from build123d import *

# Parameters (mm, degrees)
SKETCH1_R           = 25
BOSS_EXTRUDE1_DEPTH = 10
FILLET1_R           = 10
BOSS_EXTRUDE2_DEPTH = 3.6
SKETCH3_W           = 3
SKETCH3_H           = 8
BOSS_EXTRUDE3_DEPTH = 27
SKETCH4_R           = 2.4
CUT_EXTRUDE1_DEPTH  = 49.830420846
FILLET2_R           = 4
FILLET3_R           = 1


with BuildPart() as part:
    # Sketch1 → Boss-Extrude1 (new body)
    with BuildSketch(Plane(origin=(0, 0, 0), x_dir=(1, 0, 0), z_dir=(0, 1, 0))):
        with Locations(Location((0, 0, 0), (0, 0, 270))):
            Circle(SKETCH1_R)
    extrude(amount=BOSS_EXTRUDE1_DEPTH)

    # Fillet1
    fillet1_edges = [part.edges().sort_by_distance(p)[0] for p in [
        (0, 10, -25),
    ]]
    fillet(fillet1_edges, radius=FILLET1_R - 0.0001)  # a hair under: the kernel refuses the full size

    # Sketch2 → Boss-Extrude2 (add)
    with BuildSketch(Plane(origin=(0, 10, 0), x_dir=(1, 0, 0), z_dir=(0, 1, 0))):
        with BuildLine():
            Line((-2.226875614, -0.895), (-0.895, -0.895))
            Line((-0.895, -0.895), (-0.895, -2.226875614))
            ThreePointArc((-0.895, -2.226875614), (0, -2.4), (0.895, -2.226875614))
            Line((0.895, -2.226875614), (0.895, -0.895))
            Line((0.895, -0.895), (2.226875614, -0.895))
            ThreePointArc((2.226875614, -0.895), (2.4, 0), (2.226875614, 0.895))
            Line((2.226875614, 0.895), (0.895, 0.895))
            Line((0.895, 0.895), (0.895, 2.226875614))
            ThreePointArc((0.895, 2.226875614), (0, 2.4), (-0.895, 2.226875614))
            Line((-0.895, 2.226875614), (-0.895, 0.895))
            Line((-0.895, 0.895), (-2.226875614, 0.895))
            ThreePointArc((-2.226875614, 0.895), (-2.4, 0), (-2.226875614, -0.895))
        make_face()
    extrude(amount=BOSS_EXTRUDE2_DEPTH)

    # Sketch3 → Boss-Extrude3 (add)
    with BuildSketch(Plane.XZ):
        with Locations((-5.6, 0)):
            Rectangle(SKETCH3_W, SKETCH3_H)
        with Locations((5.6, 0)):
            Rectangle(SKETCH3_W, SKETCH3_H)
    extrude(amount=-BOSS_EXTRUDE3_DEPTH)

    # Sketch4 → Cut-Extrude1 (cut, through all)
    with BuildSketch(Plane(origin=(7.1, 0, 0), x_dir=(0, 0, -1), z_dir=(1, 0, 0))):
        with Locations((0, 23)):
            Circle(SKETCH4_R)
    extrude(amount=-CUT_EXTRUDE1_DEPTH, mode=Mode.SUBTRACT)

    # Fillet2
    fillet2_edges = [part.edges().sort_by_distance(p)[0] for p in [
        (5.6, 27, -4),
        (5.6, 27, 4),
        (-5.6, 27, 4),
        (-5.6, 27, -4),
    ]]
    fillet(fillet2_edges, radius=FILLET2_R - 0.0001)  # a hair under: the kernel refuses the full size

    # Fillet3
    fillet3_edges = [part.edges().sort_by_distance(p)[0] for p in [
        (-7.1, 10, 0),
        (-5.6, 10, 4),
        (-5.6, 10, -4),
        (5.6, 10, 4),
        (7.1, 10, 0),
        (5.6, 10, -4),
    ]]
    fillet(fillet3_edges, radius=FILLET3_R)


solid = part.part
Verification items for the finished model (mm, model axes). A direction names the side the tool comes from. Give positions to 0.01 mm unless a question says otherwise; leave off trailing zeros. Write each loop counter-clockwise with the first axis right and the second up, starting at its lowest first coordinate (ties: lowest second). Pieces come first, ordered by that corner, then holes. Notation, with made-up numbers: M 81,49.5 L 132,49.5 A10 ccw 132,65.5 Z; hole C 39.5,26 d1. An arc over 180 degrees is marked long. Put each result on its own line as item: value. Start each with the question number.
1. Draft check along X on faces 1 (the face through (5.621, 25.797, -2.859)), 2 (the face through (2, 12, -0.895)), 3 (the face through (-2, 12, -0.895)). Enter one of: +X half, -X half, draft (parallel to the pull), parting line (faces both ways), or undercut.
2. Section check C-C (y = 2). Record the cut outline in (x, z), and give its area (3 significant figures).
3. Scan lines: line 1 along Y through (x, z) = (-5, 0); line 2 along X through (y, z) = (14, 2.5); line 3 along Y through (x, z) = (11.5, -2). Record each from-to range of solid material in increasing order. Write a range as [from, to].
4. Section check A-A (y = 18.5). Record the cut outline in (x, z).
5. Go/stop test with flat-tipped pins: pin 1 Ø1 at (x, z) = (7, -16.5) entering from +Y; pin 2 Ø0.9 at (x, y) = (-6, 20) entering from +Z; pin 3 Ø1.1 at (x, y) = (-1.5, 11) entering from +Z (3 decimals). Record where each tip stops, or that it passes through.
6. Set-up check for faces 4 (the face through (0.895, 12, -2)), 5 (the face through (0, 11.8, 2.4)), 6 (the face through (-4.1, 16, 0)), 7 (the face through (2.4, 11.8, 0)), 8 (the face through (-6, 17, 4)): record each of +Z, -Z, +X, -X, +Y, -Y from which the full face is reachable in a straight line by a thin tool's end or side.
Answer list:
1. face 1: draft
1. face 2: undercut
1. face 3: undercut
2. outline: C 0,0 d49.6
2. area: 1,930 mm2
3. line 1: [0, 20.6], [25.4, 27]
3. line 2: [-7.1, -4.1], [4.1, 7.1]
3. line 3: [0, 10]
4. outline: M -7.1,-4 L -4.1,-4 L -4.1,4 L -7.1,4 Z; M 4.1,-4 L 7.1,-4 L 7.1,4 L 4.1,4 Z
5. pin 1: y = 9.7
5. pin 2: z = 4
5. pin 3: z = 0.895
6. face 4: -Z, +Y
6. face 5: +Z, +Y
6. face 6: +Z, -Z, +Y
6. face 7: +Y
6. face 8: +Z, +X, -X, +Y
